Geometry check sheet. Reference: drawing and pictorial views, mm from the part's lowest x, y, z. A direction names the side the tool comes from. Round coordinates to 2 decimals unless told otherwise and drop trailing zeros. Write each loop counter-clockwise with the first axis right and the second up, starting at its lowest first coordinate (ties: lowest second). Pieces come first, ordered by that corner, then holes. Notation, with made-up numbers: (-4.75, 29) -> (15.25, 29) arc R15 ccw to (15.25, 38) -> close; hole circle Ø11 at (40, -25.5). An arc over 180 degrees is marked (long way). Answer as a JSON object with one key per item and string values. Group by question number.
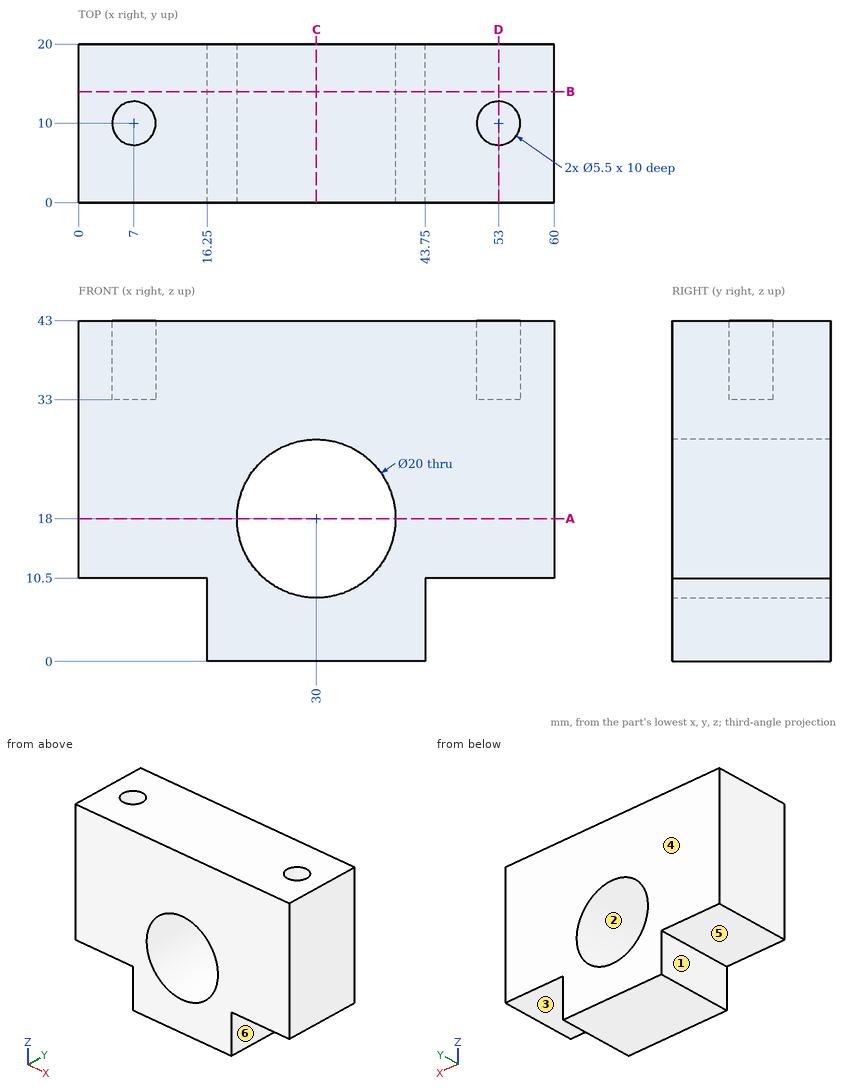
(1) Access from +Z, -Z, +X, -X, +Y, -Y to the whole of each face (thin tool, end or side, straight path). Record for the marked faces 4, 5 and 6.
(2) Go/stop test with flat-tipped pins: pin 1 Ø8 at (x, y) = (49.5, 13.5) entering from -Z; pin 2 Ø12 at (x, z) = (27.5, 20.5) entering from +Y; pin 3 Ø3 at (y, z) = (15, 4) entering from -X; pin 4 Ø3 at (y, z) = (11, 4) entering from +X. Record where each tip stops, or that it passes through.
(3) Section check B-B on y = 14. Record the cut outline in (x, z), then the cut area to 3 significant figures.
(4) Section check D-D on x = 53. Record the cut outline in (y, z).
(5) Section check C-C on x = 30. Record the cut outline in (y, z), then the cut area to 3 significant figures.
(6) Release check for a two-part mould opening along X. For the marked faces 1, 2 and 3 record: pulls with the +X half, pulls with the -X half, needs draft (parallel to the pull), parting line crosses it, or undercut.
(7) Scan lines: line 1 along X through (y, z) = (5.5, 18); line 2 along Y through (x, z) = (7, 36.75); line 3 along Z through (x, y) = (11.5, 8.25). Record each from-to range of solid material in increasing order.
(8) Section check A-A on z = 18. Record the cut outline in (x, y), then the cut area to 3 significant figures.
Data:
{
 "1": {"face 4": "+Z, -Z, +X, -X, +Y", "face 5": "-Z, -X, +Y, -Y", "face 6": "-Z, +X, +Y, -Y"},
 "2": {"pin 1": "stops at z = 10.5", "pin 2": "passes through", "pin 3": "stops at x = 16.25", "pin 4": "stops at x = 43.75"},
 "3": {"outline": "(0, 10.5) -> (16.25, 10.5) -> (16.25, 0) -> (43.75, 0) -> (43.75, 10.5) -> (60, 10.5) -> (60, 43) -> (0, 43) -> close; hole circle Ø20 at (30, 18)", "area": "1,920 mm²"},
 "4": {"outline": "(0, 10.5) -> (20, 10.5) -> (20, 43) -> (12.75, 43) -> (12.75, 33) -> (7.25, 33) -> (7.25, 43) -> (0, 43) -> close"},
 "5": {"outline": "(0, 0) -> (20, 0) -> (20, 8) -> (0, 8) -> close; (0, 28) -> (20, 28) -> (20, 43) -> (0, 43) -> close", "area": "460 mm²"},
 "6": {"face 1": "pulls with the -X half", "face 2": "undercut", "face 3": "needs draft"},
 "7": {"line 1": "x = 0 to 20, 40 to 60", "line 2": "y = 0 to 7.25, 12.75 to 20", "line 3": "z = 10.5 to 43"},
 "8": {"outline": "(0, 0) -> (20, 0) -> (20, 20) -> (0, 20) -> close; (40, 0) -> (60, 0) -> (60, 20) -> (40, 20) -> close", "area": "800 mm²"}
}
